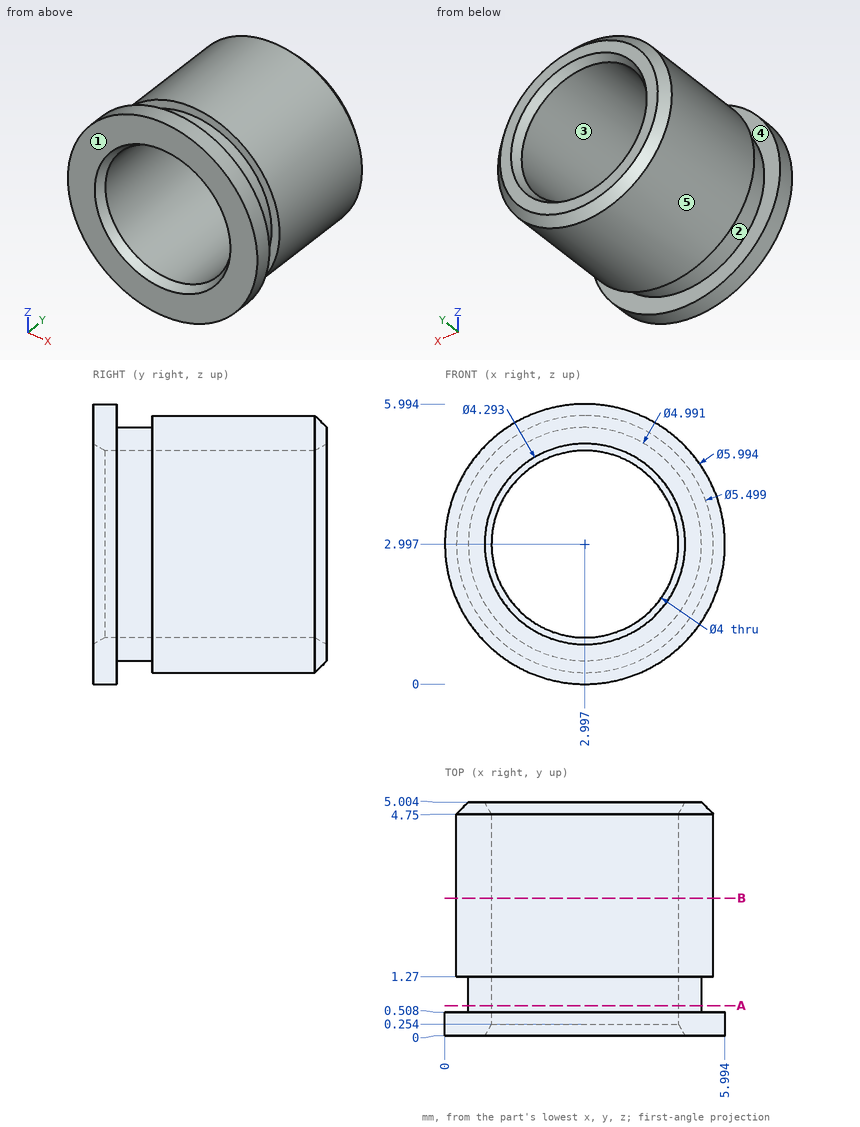
Check sheet for the drawn part. Datum: minimum x, y, z corner. Units: mm. A direction names the side the tool comes from. Give positions to 0.01 mm unless a question says otherwise; leave off trailing zeros. Order: outer loops, then holes, each group sorted by start corner. A loop starts at its lowest first (then second) coordinate and runs counter-clockwise, first axis right, second up. Notation, with made-up numbers: (11, 74.25) - (26, 74.25) arc R5 cw to (26, 78.25) - close; hole circle Ø6 at (69, 84.25). An arc over 180 degrees is marked (long way). Answer in a Markdown table with one row per item. Add a question column.
Q1. Gauge pin test, flat ends, axial feed: pin 1 (1 mm diameter, centred on x = 1.5, z = 2.5, fed in from +Y) (1 decimal); pin 2 (2 mm diameter, centred on x = 2.5, y = 2.5, fed in from -Z); pin 3 (2 mm diameter, centred on y = 4, z = 2, fed in from +X). Record the tip position at first contact, or that the pin passes through.
Q2. Material ranges on probe 1 along X at (y, z) = (3.15, 3); probe 2 along X at (y, z) = (4.6, 4.1) (1 decimal); probe 3 along Z at (x, y) = (1.8, 2.65) (1 decimal), recorded low to high. Write a range as from..to.
Q3. Cross-section at A-A, the plane y = 0.65. Enter the section's corners in (x, z) (1 decimal).
Q4. Mould release check, pull along X, two halves, no side actions. Record for the marked faces 1, 2 and 3: pulls with the +X half, pulls with the -X half, needs draft (parallel to the pull), parting line crosses it, or undercut.
Q5. Tool access check on the marked faces 4 and 5. Record the directions out of +Z, -Z, +X, -X, +Y, -Y that give a thin tool (end or side, any length) a straight path to the whole face; none if there is none.
Q6. Cross-section at B-B, the plane y = 2.95. Enter the section's corners in (x, z), then the cut area to 3 significant figures.
Check values:
| question | item | result |
|---|---|---|
| 1 | pin 1 | stops at y = 4.9 |
| 1 | pin 2 | stops at z = 0.25 |
| 1 | pin 3 | stops at x = 5.75 |
| 2 | probe 1 | x = 0.25..1, 5..5.75 |
| 2 | probe 2 | x = 0.5..1.3, 4.7..5.5 |
| 2 | probe 3 | z = 0.5..1.4, 4.6..5.5 |
| 3 | outline | circle Ø5 at (3, 3); hole circle Ø4 at (3, 3) |
| 4 | face 1 | needs draft |
| 4 | face 2 | parting line crosses it |
| 4 | face 3 | undercut |
| 5 | face 4 | none |
| 5 | face 5 | +Y |
| 6 | outline | circle Ø5.5 at (3, 3); hole circle Ø4 at (3, 3) |
| 6 | area | 11.2 mm^2 |
